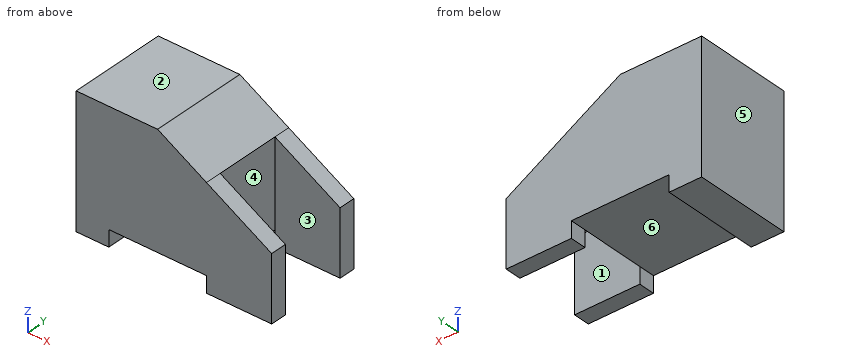
from build123d import *

# Parameters (mm, degrees)
F1_DEPTH = 7.5
F2_DEPTH = 5


with BuildPart() as f1:
    # F0 (on Front) → F1 (new body, symmetric)
    with BuildSketch(Plane.XZ):
        Polygon((0, 20), (0, 0), (5, 0), (5, 2.5), (20, 2.5), (20, 15.714286), (12.5, 20), align=None)
        Polygon((30, 10), (20, 15.714286), (20, 2.5), (20, 0), (30, 0), align=None)
    extrude(amount=F1_DEPTH, both=True)

    # F0 (on Front) → F2 (cut, symmetric)
    with BuildSketch(Plane.XZ):
        Polygon((30, 10), (20, 15.714286), (20, 2.5), (20, 0), (30, 0), align=None)
    extrude(amount=F2_DEPTH, both=True, mode=Mode.SUBTRACT)


solid = f1.part
Input: part model. Units: mm. Frame: model coordinates. Face numbers are marked on the shaded views. A direction names the side the tool comes from. Give positions to 0.01 mm unless a question says otherwise; leave off trailing zeros. Write each loop counter-clockwise with the first axis right and the second up, starting at its lowest first coordinate (ties: lowest second). Pieces come first, ordered by that corner, then holes. Notation, with made-up numbers: (64.25, 74.5) -> (101.25, 74.5) arc R22 cw to (101.25, 86.5) -> close; hole circle Ø5 at (88.5, -39). An arc over 180 degrees is marked (long way). Use one line per item in the form item = value. Start each with the question number.
1) Section query C-C on x = 11.25. Return the cut outline in (y, z), then the cut area to 4 significant figures.
2) Ray query, probe 1 along Y at (x, z) = (25, 1); probe 2 along X at (y, z) = (3.5, 13.75); probe 3 along X at (y, z) = (-1.5, 1.75). Return the intervals inside material, ascending. Write a range as from..to.
3) Section query A-A on z = 7.5. Return the cut outline in (x, y), then the cut area to 3 significant figures.
4) Set-up query: the marked faces 1 and 2. Return all of +Z, -Z, +X, -X, +Y, -Y with unobstructed straight access to the full face (end or side cutting, diameter ignored); none if empty.
5) Draft query along X for the marked faces 3, 4, 5 and 6. Return one class per face: pulls with the +X half, pulls with the -X half, needs draft (parallel to the pull), parting line crosses it, or undercut.
6) Section query B-B on y = -6.5. Return the cut outline in (x, z).
7) Section query D-D on y = -1.25. Return the cut outline in (x, z).
8) Pin query (flat end, axial travel): pin 1 (1.2 mm diameter, centred on y = 6, z = 1.5, fed in from -X); pin 2 (3 mm diameter, centred on x = 14, y = 5.5, fed in from -Z); pin 3 (3 mm diameter, centred on y = -0.5, z = 0.5, fed in from +X). Return the tip coordinate at first contact, or that it passes through.
Outcome:
q1.outline = (-7.5, 2.5) -> (7.5, 2.5) -> (7.5, 20) -> (-7.5, 20) -> close
q1.area = 262.5 mm^2
q2.probe_1 = -7.5..-5, 5..7.5
q2.probe_2 = 0..20
q2.probe_3 = 0..5
q3.outline = (0, -7.5) -> (30, -7.5) -> (30, -5) -> (20, -5) -> (20, 5) -> (30, 5) -> (30, 7.5) -> (0, 7.5) -> close
q3.area = 350 mm^2
q4.face_1 = +Z, -Z, +X
q4.face_2 = +Z, +X, -X, +Y, -Y
q5.face_3 = needs draft
q5.face_4 = pulls with the +X half
q5.face_5 = pulls with the -X half
q5.face_6 = undercut
q6.outline = (0, 0) -> (5, 0) -> (5, 2.5) -> (20, 2.5) -> (20, 0) -> (30, 0) -> (30, 10) -> (12.5, 20) -> (0, 20) -> close
q7.outline = (0, 0) -> (5, 0) -> (5, 2.5) -> (20, 2.5) -> (20, 15.71) -> (12.5, 20) -> (0, 20) -> close
q8.pin_1 = 0
q8.pin_2 = 2.5
q8.pin_3 = 5
